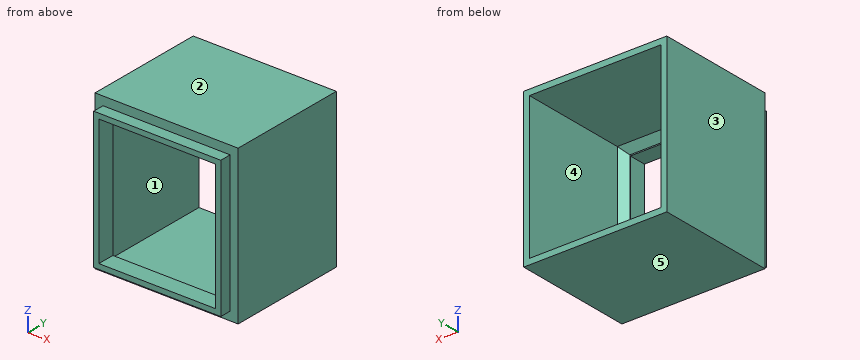
```python
from build123d import *

# Parameters (mm, degrees)
SKETCH1_W           = 111
SKETCH1_H           = 120
SKETCH1_W_2         = 102
SKETCH1_H_2         = 111
BOSS_EXTRUDE1_DEPTH = 10
SKETCH2_W           = 125
SKETCH2_H           = 135
SKETCH2_W_2         = 102
SKETCH2_H_2         = 111
BOSS_EXTRUDE2_DEPTH = 5
SKETCH4_W           = 125
SKETCH4_H           = 135
SKETCH4_W_2         = 115
SKETCH4_H_2         = 125
BOSS_EXTRUDE4_DEPTH = 100
CHAMFER1_SIZE       = 6


with BuildPart() as part:
    # Sketch1 → Boss-Extrude1 (new body)
    with BuildSketch(Plane(origin=(0, 0, 0), x_dir=(1, 0, 0), z_dir=(0, 1, 0))):
        Rectangle(SKETCH1_W, SKETCH1_H)
        Rectangle(SKETCH1_W_2, SKETCH1_H_2, mode=Mode.SUBTRACT)
    extrude(amount=BOSS_EXTRUDE1_DEPTH)

    # Sketch2 → Boss-Extrude2 (add)
    with BuildSketch(Plane(origin=(0, 10, 0), x_dir=(1, 0, 0), z_dir=(0, 1, 0))):
        Rectangle(SKETCH2_W, SKETCH2_H)
        Rectangle(SKETCH2_W_2, SKETCH2_H_2, mode=Mode.SUBTRACT)
    extrude(amount=BOSS_EXTRUDE2_DEPTH)

    # Sketch4 → Boss-Extrude4 (add)
    with BuildSketch(Plane(origin=(0, 15, 0), x_dir=(1, 0, 0), z_dir=(0, 1, 0))):
        Rectangle(SKETCH4_W, SKETCH4_H)
        Rectangle(SKETCH4_W_2, SKETCH4_H_2, mode=Mode.SUBTRACT)
    extrude(amount=BOSS_EXTRUDE4_DEPTH)

    # Chamfer1
    chamfer1_edges = [part.edges().sort_by_distance(p)[0] for p in [
        (0, 15, -62.5),
        (-57.5, 15, 0),
        (0, 15, 62.5),
        (57.5, 15, 0),
    ]]
    chamfer(chamfer1_edges, length=CHAMFER1_SIZE)


solid = part.part
```
The listing builds one solid part. Answer for the finished solid, in the listing's coordinates (mm). Face numbers are marked on the shaded views. A direction names the side the tool comes from. Give positions to 0.01 mm unless a question says otherwise; leave off trailing zeros. Order: outer loops, then holes, each group sorted by start corner. A loop starts at its lowest first (then second) coordinate and runs counter-clockwise, first axis right, second up. Notation, with made-up numbers: (42, 88.5) -> (52, 88.5) arc R21 cw to (52, 119.5) -> close; hole circle Ø2 at (-4, 36). An arc over 180 degrees is marked (long way). Answer as a JSON object with one key per item and string values. Group by question number.
Item 1: The part is cut by section B-B on z = -5. Write down the section's boundary in (x, y).
Item 2: Consider L1, parallel to Z at x = 18, y = 85; L2, parallel to X at y = 72, z = 2; L3, parallel to X at y = 20.5, z = 6. Determine where each line is inside the solid, lowest interval first. Write a range as from..to.
Item 3: The part is cut by section A-A on y = 51. Write down the section's boundary in (x, z).
Item 4: Flat-ended cylindrical pins translate along their axes: pin 1 (5 mm diameter, centred on x = -20, y = 4, fed in from -Z); pin 2 (5 mm diameter, centred on y = 2.5, z = -3.5, fed in from +X); pin 3 (11 mm diameter, centred on y = 4, z = -19, fed in from -X); pin 4 (5 mm diameter, centred on x = -3.5, z = -52.5, fed in from -Y). Find the tip coordinate at first contact, or state that the pin passes through.
Item 5: The part is cut by section C-C on x = 28. Write down the section's boundary in (y, z).
Item 6: A tool of negligible diameter and unlimited length cuts with its end or side. For the marked faces 4 and 5, from which of +Z, -Z, +X, -X, +Y, -Y can it reach the whole face along a straight path? Write none if from no direction.
Item 7: Determine the mould class of the marked faces 1, 2 and 3 for opening direction Z: pulls with the +Z half, pulls with the -Z half, needs draft (parallel to the pull), parting line crosses it, or undercut.
Result set:
{
 "1": {"outline": "(-62.5, 10) -> (-55.5, 10) -> (-55.5, 0) -> (-51, 0) -> (-51, 15) -> (-51.5, 15) -> (-57.5, 21) -> (-57.5, 115) -> (-62.5, 115) -> close; (51, 0) -> (55.5, 0) -> (55.5, 10) -> (62.5, 10) -> (62.5, 115) -> (57.5, 115) -> (57.5, 21) -> (51.5, 15) -> (51, 15) -> close"},
 "2": {"L1": "-67.5..-62.5, 62.5..67.5", "L2": "-62.5..-57.5, 57.5..62.5", "L3": "-62.5..-57, 57..62.5"},
 "3": {"outline": "(-62.5, -67.5) -> (62.5, -67.5) -> (62.5, 67.5) -> (-62.5, 67.5) -> close; hole (-57.5, -62.5) -> (57.5, -62.5) -> (57.5, 62.5) -> (-57.5, 62.5) -> close"},
 "4": {"pin 1": "z = -60", "pin 2": "x = 55.5", "pin 3": "x = -55.5", "pin 4": "through"},
 "5": {"outline": "(0, -60) -> (10, -60) -> (10, -67.5) -> (115, -67.5) -> (115, -62.5) -> (21, -62.5) -> (15, -56.5) -> (15, -55.5) -> (0, -55.5) -> close; (0, 55.5) -> (15, 55.5) -> (15, 56.5) -> (21, 62.5) -> (115, 62.5) -> (115, 67.5) -> (10, 67.5) -> (10, 60) -> (0, 60) -> close"},
 "6": {"face 4": "+Y", "face 5": "-Z, +X, -X, +Y, -Y"},
 "7": {"face 1": "undercut", "face 2": "pulls with the +Z half", "face 3": "needs draft"}
}
